```python
from build123d import *

# Parameters (mm, degrees)
NORTH_SOUTH_SKETCH_R              = 5
NORTH_SOUTH_EXTRUDE_DEPTH         = 60
EAST_WEST_EXTRUDE_DEPTH           = 30
EAST_WEST_EXTRUDE_DEPTH_BACK      = 30
EAST_WEST_SKETCH_R                = 5
CENTER_SUPPORT_EXTRUDE_DEPTH      = 5
CENTER_SUPPORT_EXTRUDE_DEPTH_BACK = 5
CENTER_SUPPORT_SKETCH_R           = 15


with BuildPart() as part:
    # North-South Sketch → North-South Extrude (new body)
    with BuildSketch(Plane.XY):
        Circle(NORTH_SOUTH_SKETCH_R)
    extrude(amount=NORTH_SOUTH_EXTRUDE_DEPTH)

    # East-West Sketch → East-West Extrude (add, two sides: drawn at the far end of the back side and taken through both)
    with BuildSketch(Plane(origin=(0, 0, 0), x_dir=(0, 0, -1), z_dir=(1, 0, 0)).offset(-EAST_WEST_EXTRUDE_DEPTH_BACK)):
        with Locations((-30, 0)):
            Circle(EAST_WEST_SKETCH_R)
    extrude(amount=EAST_WEST_EXTRUDE_DEPTH + EAST_WEST_EXTRUDE_DEPTH_BACK)

    # Center Support Sketch → Center Support Extrude (add, two sides: drawn at the far end of the back side and taken through both)
    with BuildSketch(Plane(origin=(0, 0, 0), x_dir=(1, 0, 0), z_dir=(0, 1, 0)).offset(-CENTER_SUPPORT_EXTRUDE_DEPTH_BACK)):
        with Locations((0, -30)):
            Circle(CENTER_SUPPORT_SKETCH_R)
    extrude(amount=CENTER_SUPPORT_EXTRUDE_DEPTH + CENTER_SUPPORT_EXTRUDE_DEPTH_BACK)


solid = part.part
```
The listing builds one solid part. Answer for the finished solid, in the listing's coordinates (mm). A direction names the side the tool comes from. Coordinates: 2 decimals unless noted, no trailing zeros. Write each loop counter-clockwise with the first axis right and the second up, starting at its lowest first coordinate (ties: lowest second). Pieces come first, ordered by that corner, then holes. Notation, with made-up numbers: (-18, 13) - (-8, 13) arc R19 cw to (-8, 43) - close; hole circle Ø5 at (-38.5, 16.25). An arc over 180 degrees is marked (long way). Return JSON: item names as keys, results as strings. Group by question number.
Q1. The part is cut by section D-D on y = 3. Write down the section's boundary in (x, z), and give its area (3 significant figures).
Q2. The part is cut by section A-A on y = 0. Write down the section's boundary in (x, z).
Q3. Find the intervals of material crossed by line 1 along X through (y, z) = (2, 35); line 2 along X through (y, z) = (0, 6.5); line 3 along Z through (x, y) = (26, 0.75), in increasing order. Write a range as [from, to].
Q4. The part is cut by section B-B on z = 33. Write down the section's boundary in (x, y).
Q5. Flat-ended cylindrical pins translate along their axes: pin 1 Ø1.5 at (y, z) = (0.5, 38.5) entering from +X; pin 2 Ø5 at (x, y) = (23, 2) entering from -Z; pin 3 Ø1.5 at (x, y) = (-22, -1) entering from +Z. Find the tip coordinate at first contact, or state that the pin passes through.
Q6. Which of the six approach directions +Z, -Z, +X, -X, +Y, -Y give full straight-line access (tool end or side, diameter ignored) to faces 1 (the cylindrical face through (-22, 0, 35)), 2 (the cylindrical face through (-1.08, -4.88, 7.82)), 3 (the cylindrical face through (4.77, 1.5, 51.96))?
Q7. The part is cut by section C-C on x = 7.5. Write down the section's boundary in (y, z), and give its area (3 significant figures).
Evaluation:
{
 "1": {"outline": "(-30, 26) - (-14.46, 26) arc R15 ccw to (-4, 15.54) - (-4, 0) - (4, 0) - (4, 15.54) arc R15 ccw to (14.46, 26) - (30, 26) - (30, 34) - (14.46, 34) arc R15 ccw to (4, 44.46) - (4, 60) - (-4, 60) - (-4, 44.46) arc R15 ccw to (-14.46, 34) - (-30, 34) - close", "area": "1,190 mm2"},
 "2": {"outline": "(-30, 25) - (-14.14, 25) arc R15 ccw to (-5, 15.86) - (-5, 0) - (5, 0) - (5, 15.86) arc R15 ccw to (14.14, 25) - (30, 25) - (30, 35) - (14.14, 35) arc R15 ccw to (5, 44.14) - (5, 60) - (-5, 60) - (-5, 44.14) arc R15 ccw to (-14.14, 35) - (-30, 35) - close"},
 "3": {"line 1": "x = [-14.14, 14.14]", "line 2": "x = [-5, 5]", "line 3": "z = [25.06, 34.94]"},
 "4": {"outline": "(-30, -4) - (-14.7, -4) - (-14.7, -5) - (14.7, -5) - (14.7, -4) - (30, -4) - (30, 4) - (14.7, 4) - (14.7, 5) - (-14.7, 5) - (-14.7, 4) - (-30, 4) - close"},
 "5": {"pin 1": "stops at x = 12.84", "pin 2": "stops at z = 25", "pin 3": "stops at z = 34.99"},
 "6": {"face 1": "-X", "face 2": "-Z", "face 3": "+Z"},
 "7": {"outline": "(-5, 17.01) - (5, 17.01) - (5, 42.99) - (-5, 42.99) - close", "area": "260 mm2"}
}
